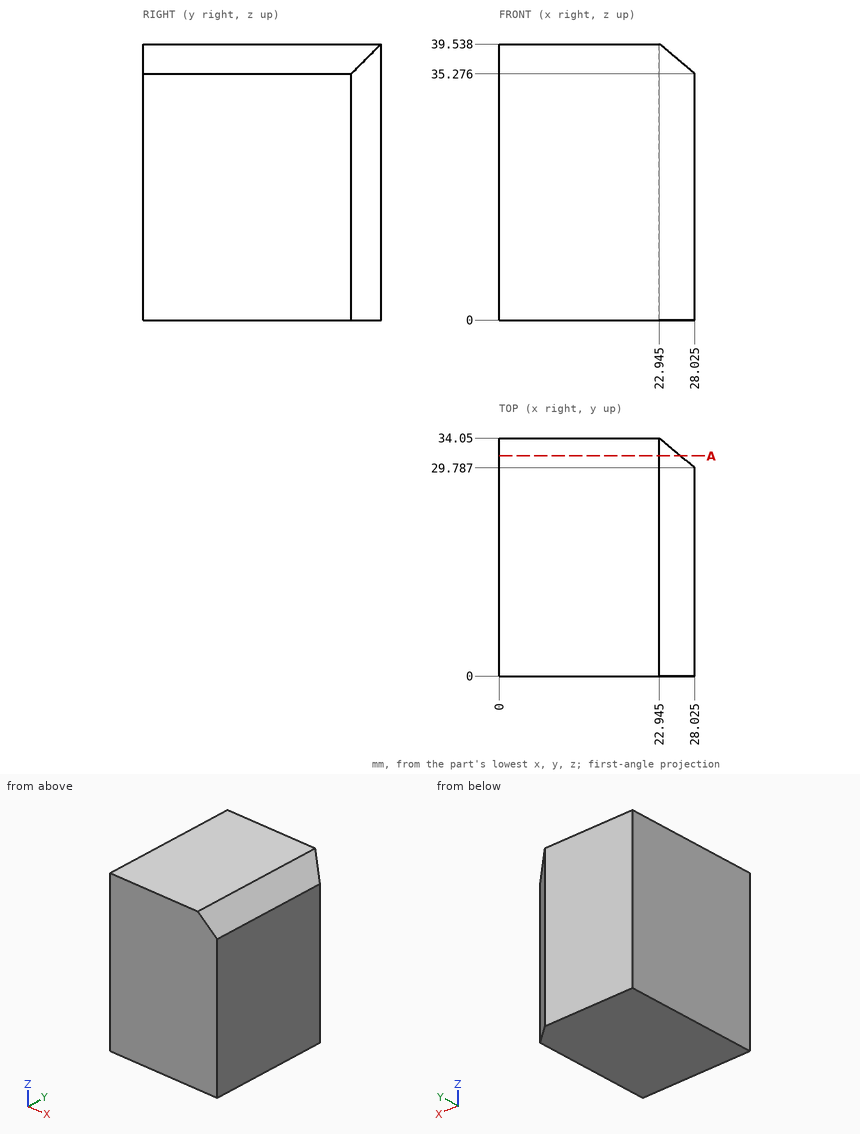
The drawing under review shows one solid part. Ordinate dimensions are in mm from its lowest x, y, z. Coordinates: 2 decimals unless noted, no trailing zeros. Order: outer loops, then holes, each group sorted by start corner. A loop starts at its lowest first (then second) coordinate and runs counter-clockwise, first axis right, second up. Notation, with made-up numbers: (40, -31.75) -> (95, -31.75) arc R29 cw to (95, 1.25) -> close; hole circle Ø6 at (-29, 16.25). An arc over 180 degrees is marked (long way). One line per item, written item: value.
1) To check wall thickness, follow probe 1 along Y at (x, z) = (25.5, 34) (1 decimal); probe 2 along X at (y, z) = (31, 2.5); probe 3 along Z at (x, y) = (25, 29.5) (1 decimal). State the ranges of each line that lie inside material, in increasing order. Write a range as [from, to].
Output values:
probe 1: y = [0, 31.9]
probe 2: x = [0, 26.58]
probe 3: z = [0, 37.8]
2) Clearance check with a flat-ended pin moving along its axis: P1, Ø4, axis at y = 12, z = 18.5, coming from the -X side. State where the tip first meets the part, or that it passes through.
Output values:
P1: stops at x = 0
3) We need section A-A, the plane y = 31.5. Give the boundary of the cut face in (x, z) (1 decimal), then the cut area to 3 significant figures.
Output values:
outline: (0, 0) -> (26, 0) -> (26, 37) -> (22.9, 39.5) -> (0, 39.5) -> close
area: 1,020 mm2
